Work out the finished part from the listing and answer in its coordinate system (mm). Face numbers are marked on the shaded views. A direction names the side the tool comes from. Coordinates: 2 decimals unless noted, no trailing zeros. Order: outer loops, then holes, each group sorted by start corner. A loop starts at its lowest first (then second) coordinate and runs counter-clockwise, first axis right, second up. Notation, with made-up numbers: (20, 20.25) - (31, 20.25) arc R17 ccw to (31, 41.25) - close; hole circle Ø11 at (66, 46.5). An arc over 180 degrees is marked (long way). Use CSV: the item, a comma, the result in double quotes. Start each with the question number.
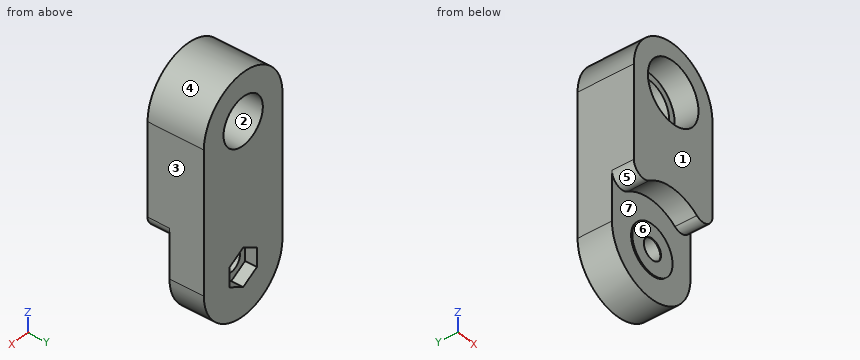
from build123d import *

# Parameters (mm, degrees)
SKETCH1_R           = 5.15
BOSS_EXTRUDE1_DEPTH = 4
SKETCH2_R           = 4
BOSS_EXTRUDE2_DEPTH = 5.5
SKETCH3_R           = 8.25
CUT_EXTRUDE1_DEPTH  = 3.7
CUT_EXTRUDE2_REACH  = 7.8
SKETCH4_R           = 1.75
SKETCH5_R           = 4.1
SKETCH5_R_2         = 1.75
BOSS_EXTRUDE3_DEPTH = 0.2
CUT_EXTRUDE3_DEPTH  = 2
FILLET1_R           = 2


with BuildPart() as part:
    # Sketch1 → Boss-Extrude1 (new body)
    with BuildSketch(Plane(origin=(0, 0, 0), x_dir=(1, 0, 0), z_dir=(0, 1, 0))):
        with BuildLine():
            Line((-8, 23.95), (-8, 0))
            ThreePointArc((-8, 0), (0, -8), (8, 0))
            Line((8, 0), (8, 23.95))
            ThreePointArc((8, 23.95), (0, 31.95), (-8, 23.95))
        make_face()
        Circle(SKETCH1_R, mode=Mode.SUBTRACT)
    extrude(amount=BOSS_EXTRUDE1_DEPTH)

    # Sketch2 → Boss-Extrude2 (add)
    with BuildSketch(Plane(origin=(0, 4, 0), x_dir=(1, 0, 0), z_dir=(0, 1, 0))):
        with BuildLine():
            Line((-8, 23.95), (-8, 0))
            ThreePointArc((-8, 0), (0, -8), (8, 0))
            Line((8, 0), (8, 23.95))
            ThreePointArc((8, 23.95), (0, 31.95), (-8, 23.95))
        make_face()
        Circle(SKETCH2_R, mode=Mode.SUBTRACT)
    extrude(amount=BOSS_EXTRUDE2_DEPTH)

    # Sketch3 → Cut-Extrude1 (cut)
    with BuildSketch(Plane(origin=(0, 0, 0), x_dir=(1, 0, 0), z_dir=(0, 1, 0))):
        with Locations((0, 23.95)):
            Circle(SKETCH3_R)
    extrude(amount=CUT_EXTRUDE1_DEPTH, mode=Mode.SUBTRACT)

    # Sketch4 → Cut-Extrude2 (cut, up to next)
    with BuildSketch(Plane.XZ.offset(-3.7), mode=Mode.PRIVATE) as cut_extrude2_sk1:
        with Locations((0, -23.95)):
            Circle(SKETCH4_R)
    cut_extrude2_tool1 = extrude(cut_extrude2_sk1.sketch, amount=-CUT_EXTRUDE2_REACH, mode=Mode.PRIVATE) & part.part
    add(cut_extrude2_tool1.solids().sort_by_distance((0, 3.7, -23.95))[0], mode=Mode.SUBTRACT)

    # Sketch5 → Boss-Extrude3 (add)
    with BuildSketch(Plane.XZ.offset(-3.7)):
        with Locations((0, -23.95)):
            Circle(SKETCH5_R)
        with Locations((0, -23.95)):
            Circle(SKETCH5_R_2, mode=Mode.SUBTRACT)
    extrude(amount=BOSS_EXTRUDE3_DEPTH)

    # Sketch6 → Cut-Extrude3 (cut)
    with BuildSketch(Plane(origin=(0, 9.5, 0), x_dir=(1, 0, 0), z_dir=(0, 1, 0))):
        Polygon((0, 20.716838493), (2.8, 22.333419246), (2.8, 25.566580754), (0, 27.183161507), (-2.8, 25.566580754), (-2.8, 22.333419246), align=None)
    extrude(amount=-CUT_EXTRUDE3_DEPTH, mode=Mode.SUBTRACT)

    # Fillet1
    fillet1_edges = [part.edges().sort_by_distance(p)[0] for p in [
        (8, 1.85, -21.934435563),
        (-8, 1.85, -21.934435563),
    ]]
    fillet(fillet1_edges, radius=FILLET1_R)


solid = part.part
1) For the marked faces 4, 5, 6 and 7, determine the directions among +Z, -Z, +X, -X, +Y, -Y from which every point of the face is accessible in a straight line to the end or side of a thin tool.
2) Straight lines are drawn through the part: line 1 (Z direction, x = 0, y = 7.2); line 2 (Z direction, x = 0, y = 8.3); line 3 (Y direction, x = 1.5, z = -23). For each, find the intervals that lie inside material, in ascending order. Write a range as [from, to].
3) The part is cut by section A-A on y = 8.25. Determine the outline of the cut face in (x, z), plus the area to 3 significant figures.
4) The part is cut by section B-B on z = -3.5. Determine the outline of the cut face in (x, y), plus the area to 3 significant figures.
5) Flat-ended cylindrical pins translate along their axes: P1, Ø5.5, axis at x = 0, z = -23.95, coming from the +Y side; P2, Ø1.5, axis at x = -2.5, z = -19, coming from the -Y side; P3, Ø6.5, axis at x = 1.5, z = -25.5, coming from the -Y side. Find the tip coordinate at first contact, or state that the pin passes through.
6) The part is cut by section D-D on y = 2.25. Determine the outline of the cut face in (x, z).
7) For a pull along X with two mould halves and no side action, classify the marked faces 1, 2 and 3 as +X half, -X half, draft (parallel to the pull), parting line (faces both ways), or undercut.
8) The part is cut by section C-C on x = 0.75. Determine the outline of the cut face in (y, z).
Answer key:
1,face 4,"+Z, +Y, -Y"
1,face 5,"-Z, -Y"
1,face 6,"-Z, +X, -X, -Y"
1,face 7,"-Y"
2,line 1,"[-31.95, -25.7], [-22.2, -4], [4, 8]"
2,line 2,"[-31.95, -27.18], [-20.72, -4], [4, 8]"
2,line 3,"[3.5, 7.5]"
3,outline,"(-8, -23.95) arc R8 ccw to (8, -23.95) - (8, 0) arc R8 ccw to (-8, 0) - close; hole circle Ø8 at (0, 0); hole (-2.8, -25.57) - (0, -27.18) - (2.8, -25.57) - (2.8, -22.33) - (0, -20.72) - (-2.8, -22.33) - close"
3,area,"507 mm^2"
4,outline,"(-8, 0) - (-3.78, 0) - (-3.78, 4) - (-1.94, 4) - (-1.94, 9.5) - (-8, 9.5) - close; (1.94, 4) - (3.78, 4) - (3.78, 0) - (8, 0) - (8, 9.5) - (1.94, 9.5) - close"
4,area,"100 mm^2"
5,P1,"y = 7.5"
5,P2,"y = 3.7"
5,P3,"y = 3.5"
6,outline,"(-8, -15.64) arc R2 ccw to (-4.83, -17.26) arc R8.25 cw to (4.83, -17.26) arc R2 ccw to (8, -15.64) - (8, 0) arc R8 ccw to (-8, 0) - close; hole circle Ø10.3 at (0, 0)"
7,face 1,"draft"
7,face 2,"undercut"
7,face 3,"+X half"
8,outline,"(0, -15.73) - (3.7, -15.73) - (3.7, -19.92) - (3.5, -19.92) - (3.5, -22.37) - (7.5, -22.37) - (7.5, -21.15) - (9.5, -21.15) - (9.5, -3.93) - (4, -3.93) - (4, -5.1) - (0, -5.1) - close; (0, 5.1) - (4, 5.1) - (4, 3.93) - (9.5, 3.93) - (9.5, 7.96) - (0, 7.96) - close; (3.5, -27.98) - (3.7, -27.98) - (3.7, -31.91) - (9.5, -31.91) - (9.5, -26.75) - (7.5, -26.75) - (7.5, -25.53) - (3.5, -25.53) - close"
